```python
from build123d import *

# Parameters (mm, degrees)
SKETCH2_R                    = 98.425
SKETCH2_R_2                  = 1.9
SKETCH2_R_3                  = 73.025
SKETCH2_R_4                  = 66.675
BOSS_EXTRUDE1_DEPTH          = 6.35
BOSS_EXTRUDE2_START          = 63.5
SKETCH2_3_R                  = 73.025
SKETCH2_3_R_2                = 66.675
BOSS_EXTRUDE2_DEPTH          = 63.5
FILLET1_R                    = 6.35
SKETCH2_5_R                  = 1.9
CUT_EXTRUDE2_DEPTH           = 153.9941543
CHAMFER2_SIZE                = 2.032
CIRPATTERN1_COUNT            = 10
CHAMFER2_OF_CIRPATTERN1_SIZE = 2.032
CHAMFER3_SIZE                = 12.7
CHAMFER3_SIZE2               = 7.332348419


with BuildPart() as part:
    # Sketch2 → Boss-Extrude1 (new body)
    # profile 1 of 3: a face of its own
    with BuildSketch(Plane(origin=(0, 0, 0), x_dir=(1, 0, 0), z_dir=(0, 1, 0))):
        with Locations(Location((0, 0, 0), (0, 0, 270))):
            Circle(SKETCH2_R)
        with Locations((0, 88.9)):
            Circle(SKETCH2_R_2, mode=Mode.SUBTRACT)
        Circle(SKETCH2_R_3, mode=Mode.SUBTRACT)
    # profile 2 of 3: a face of its own
    with BuildSketch(Plane(origin=(0, 0, 0), x_dir=(1, 0, 0), z_dir=(0, 1, 0))):
        with Locations((0, 88.9)):
            Circle(SKETCH2_R_2)
    # profile 3 of 3: a face of its own
    with BuildSketch(Plane(origin=(0, 0, 0), x_dir=(1, 0, 0), z_dir=(0, 1, 0))):
        Circle(SKETCH2_R_3)
        with Locations(Location((0, 0, 0), (0, 0, 270))):
            Circle(SKETCH2_R_4, mode=Mode.SUBTRACT)
    extrude(amount=-BOSS_EXTRUDE1_DEPTH)

    # Sketch2_3 → Boss-Extrude2 (add)
    # profile 1 of 2: a face of its own
    with BuildSketch(Plane(origin=(0, 0, 0), x_dir=(1, 0, 0), z_dir=(0, 1, 0)).offset(BOSS_EXTRUDE2_START)):
        with Locations(Location((0, 0, 0), (0, 0, 270))):
            Circle(SKETCH2_3_R)
        with Locations(Location((0, 0, 0), (0, 0, 270))):
            Circle(SKETCH2_3_R_2, mode=Mode.SUBTRACT)
    # profile 2 of 2: a face of its own
    with BuildSketch(Plane(origin=(0, 0, 0), x_dir=(1, 0, 0), z_dir=(0, 1, 0)).offset(BOSS_EXTRUDE2_START)):
        with Locations(Location((0, 0, 0), (0, 0, 270))):
            Circle(SKETCH2_3_R)
        with Locations(Location((0, 0, 0), (0, 0, 270))):
            Circle(SKETCH2_3_R_2, mode=Mode.SUBTRACT)
    extrude(amount=-BOSS_EXTRUDE2_DEPTH)

    # Fillet1
    fillet1_edges = [part.edges().sort_by_distance(p)[0] for p in [
        (0, 0, -73.025),
    ]]
    fillet(fillet1_edges, radius=FILLET1_R)

    # Sketch2_5 → Cut-Extrude2 (cut, through all)
    with BuildSketch(Plane(origin=(0, 0, 0), x_dir=(1, 0, 0), z_dir=(0, 1, 0))):
        with Locations(Location((0, 88.9, 0), (0, 0, 270))):
            Circle(SKETCH2_5_R)
    cut_extrude2 = extrude(amount=-CUT_EXTRUDE2_DEPTH, mode=Mode.SUBTRACT)

    # Chamfer2
    chamfer2_edges = [part.edges().sort_by_distance(p)[0] for p in [
        (0, -6.35, -90.8),
    ]]
    chamfer(chamfer2_edges, length=CHAMFER2_SIZE)

    # CirPattern1: Cut-Extrude2 ×10 about axis
    cirpattern1_axis = Axis((0, 0, 0), (0, 1, 0))
    for i in range(1, CIRPATTERN1_COUNT):
        add(cut_extrude2.rotate(cirpattern1_axis, i * 360 / CIRPATTERN1_COUNT), mode=Mode.SUBTRACT)

    # Chamfer2 of CirPattern1
    chamfer2_of_cirpattern1_edges = [part.edges().sort_by_distance(p)[0] for p in [
        (-53.370900908, -6.35, -73.458743089),
        (-86.35593168, -6.35, -28.058743089),
        (-86.35593168, -6.35, 28.058743089),
        (-53.370900908, -6.35, 73.458743089),
        (0, -6.35, 90.8),
        (53.370900908, -6.35, 73.458743089),
        (86.35593168, -6.35, 28.058743089),
        (86.35593168, -6.35, -28.058743089),
        (53.370900908, -6.35, -73.458743089),
    ]]
    chamfer(chamfer2_of_cirpattern1_edges, length=CHAMFER2_OF_CIRPATTERN1_SIZE)

    # Chamfer3
    chamfer3_edges = [part.edges().sort_by_distance(p)[0] for p in [
        (0, -6.35, -66.675),
    ]]
    chamfer3_side = [part.faces().sort_by_distance(p)[0] for p in [
        (0, 28.575, -66.675),
    ]]
    chamfer(chamfer3_edges, length=CHAMFER3_SIZE, length2=CHAMFER3_SIZE2, reference=chamfer3_side[0])


solid = part.part
```
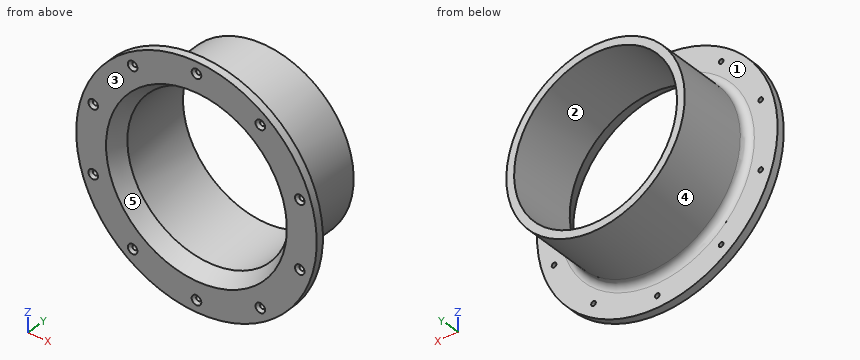
Source: CAD feature listing. Evaluate the final solid. Frame: model axes, mm. Face numbers are marked on the shaded views. A direction names the side the tool comes from. Coordinates: 2 decimals unless noted, no trailing zeros. Loops run counter-clockwise (first coordinate to the right, second up) from the corner with the lowest first, then second, coordinate; pieces in that order, holes last. Notation, with made-up numbers: M 65.5,-37 L 98.5,-37 A29 cw 98.5,1 Z; hole C 83,46 d8. An arc over 180 degrees is marked long. Use a Markdown table: item, result. Add a question column.
Q1. Access query for the marked faces 1 and 2. Directions: +Z, -Z, +X, -X, +Y, -Y. A direction counts if a zero-diameter tool reaches every point of the face in a straight line with its end or side. Return the directions, or none.
Q2. Material intervals for L1, parallel to Z at x = 48, y = 57; L2, parallel to Z at x = 56, y = 8; L3, parallel to Y at x = 76, z = 38, sorted ascending.
Q3. Section query B-B, the plane y = 30. Return loops of the section in (x, z) (3 decimals).
Q4. First-contact query: pin 1 (3.5 mm diameter, centred on x = 0, z = 88.9, fed in from +Y); pin 2 (6 mm diameter, centred on x = -47, y = 22, fed in from -Z); pin 3 (6 mm diameter, centred on x = -52.25, z = -71.92, fed in from -Y); pin 4 (2 mm diameter, centred on x = 63, y = 54, fed in from +Z). Flat tips, straight axial feed; report the tip coordinate or a pass-through.
Q5. Section query A-A, the plane z = 0. Return loops of the section in (x, y) (3 decimals).
Q6. Draft query along Z for the marked faces 3, 4 and 5. Return one class per face: pulls with the +Z half, pulls with the -Z half, needs draft (parallel to the pull), parting line crosses it, or undercut.
Result:
| question | item | result |
|---|---|---|
| 1 | face 1 | +Y |
| 1 | face 2 | +Y, -Y |
| 2 | L1 | z = -55.03 to -46.28, 46.28 to 55.03 |
| 2 | L2 | z = -46.87 to -36.19, 36.19 to 46.87 |
| 2 | L3 | y = -6.35 to 0 |
| 3 | outline | C 0,0 d146.05; hole C 0,0 d133.35 |
| 4 | pin 1 | passes through |
| 4 | pin 2 | stops at z = -58.28 |
| 4 | pin 3 | stops at y = -5.42 |
| 4 | pin 4 | stops at z = 38.58 |
| 5 | outline | M -98.425,-6.35 L -74.007,-6.35 L -66.675,6.35 L -66.675,63.5 L -73.025,63.5 L -73.025,6.35 A6.35 cw -79.375,0 L -98.425,0 Z; M 66.675,6.35 L 74.007,-6.35 L 98.425,-6.35 L 98.425,0 L 79.375,0 A6.35 cw 73.025,6.35 L 73.025,63.5 L 66.675,63.5 Z |
| 6 | face 3 | needs draft |
| 6 | face 4 | parting line crosses it |
| 6 | face 5 | undercut |
